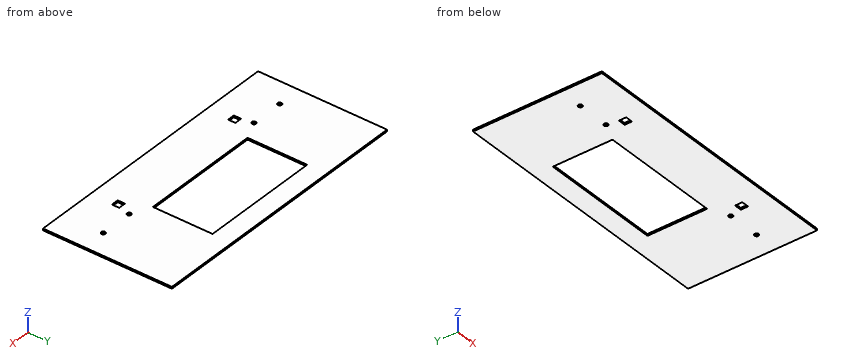
```python
from build123d import *

# Parameters (mm, degrees)
SK_PANEL_W              = 300
SK_PANEL_H              = 141.5
EX_PANEL_DEPTH          = 2
SK_DRAWEROPENING_W      = 132
SK_DRAWEROPENING_H      = 65.5
CUT_DRAWEROPENING_DEPTH = 2
SK_CLIFFBOLTS_R         = 2.25
CUT_CLIFFBOLTS_DEPTH    = 2
SK_CLIFFCABLES_W        = 8
SK_CLIFFCABLES_H        = 8
CUT_CLIFFCABLES_DEPTH   = 2


with BuildPart() as part:
    # SK_Panel → EX_Panel (new body)
    with BuildSketch(Plane.XY):
        with Locations((0, 70.75)):
            Rectangle(SK_PANEL_W, SK_PANEL_H)
    extrude(amount=EX_PANEL_DEPTH)

    # SK_DrawerOpening → CUT_DrawerOpening (cut)
    with BuildSketch(Plane.XY):
        with Locations((0, 87.25)):
            Rectangle(SK_DRAWEROPENING_W, SK_DRAWEROPENING_H)
    extrude(amount=CUT_DRAWEROPENING_DEPTH, mode=Mode.SUBTRACT)

    # SK_CliffBolts → CUT_CliffBolts (cut)
    with BuildSketch(Plane.XY):
        with Locations((123, 45)):
            Circle(SK_CLIFFBOLTS_R)
        with Locations((87, 45)):
            Circle(SK_CLIFFBOLTS_R)
        with Locations((-123, 45)):
            Circle(SK_CLIFFBOLTS_R)
        with Locations((-87, 45)):
            Circle(SK_CLIFFBOLTS_R)
    extrude(amount=CUT_CLIFFBOLTS_DEPTH, mode=Mode.SUBTRACT)

    # SK_CliffCables → CUT_CliffCables (cut)
    with BuildSketch(Plane.XY):
        with Locations((81, 28.5)):
            Rectangle(SK_CLIFFCABLES_W, SK_CLIFFCABLES_H)
        with Locations((-81, 28.5)):
            Rectangle(SK_CLIFFCABLES_W, SK_CLIFFCABLES_H)
    extrude(amount=CUT_CLIFFCABLES_DEPTH, mode=Mode.SUBTRACT)


solid = part.part
```
The listing builds one solid part. Answer for the finished solid, in the listing's coordinates (mm). Coordinates: 2 decimals unless noted, no trailing zeros. Loops run counter-clockwise (first coordinate to the right, second up) from the corner with the lowest first, then second, coordinate; pieces in that order, holes last. Notation, with made-up numbers: (80.25, 24.5) - (86.25, 24.5) arc R9 ccw to (86.25, 38.5) - close; hole circle Ø10 at (3.25, -6.75). An arc over 180 degrees is marked (long way). Write item = value, one per line.
1) Section A-A (y = 109) is taken. Determine the outline of the cut face in (x, z), plus the area to 3 significant figures.
Responses:
outline = (-150, 0) - (-66, 0) - (-66, 2) - (-150, 2) - close; (66, 0) - (150, 0) - (150, 2) - (66, 2) - close
area = 336 mm^2
2) Section B-B (x = 43) is taken. Determine the outline of the cut face in (y, z), plus the area to 3 significant figures.
Responses:
outline = (0, 0) - (54.5, 0) - (54.5, 2) - (0, 2) - close; (120, 0) - (141.5, 0) - (141.5, 2) - (120, 2) - close
area = 152 mm^2
3) Find the intervals of material crossed by line 1 along X through (y, z) = (31.5, 0.25); line 2 along X through (y, z) = (112, 1.9); line 3 along Y through (x, z) = (-12, 0.15), in increasing order.
Responses:
line_1 = -150 to -85, -77 to 77, 85 to 150
line_2 = -150 to -66, 66 to 150
line_3 = 0 to 54.5, 120 to 141.5
4) Section C-C (z = 0.35) is taken. Determine the outline of the cut face in (x, y).
Responses:
outline = (-150, 0) - (150, 0) - (150, 141.5) - (-150, 141.5) - close; hole circle Ø4.5 at (-123, 45); hole circle Ø4.5 at (-87, 45); hole (-85, 24.5) - (-77, 24.5) - (-77, 32.5) - (-85, 32.5) - close; hole (-66, 54.5) - (66, 54.5) - (66, 120) - (-66, 120) - close; hole (77, 24.5) - (85, 24.5) - (85, 32.5) - (77, 32.5) - close; hole circle Ø4.5 at (87, 45); hole circle Ø4.5 at (123, 45)
